Read the model definition and answer for the solid it produces. Units are mm, in the model's axes. A direction names the side the tool comes from. Coordinates: 2 decimals unless noted, no trailing zeros. Loops run counter-clockwise (first coordinate to the right, second up) from the corner with the lowest first, then second, coordinate; pieces in that order, holes last. Notation, with made-up numbers: (-19, 65.5) - (9, 65.5) arc R8 ccw to (9, 78.5) - close; hole circle Ø6 at (79.25, 86). An arc over 180 degrees is marked (long way). One line per question, with ' | ' between items. Start each with the question number.
```python
from build123d import *

# Parameters (mm, degrees)
SKETCH1_W           = 95.25
SKETCH1_H           = 95.25
BOSS_EXTRUDE1_DEPTH = 8.89
SKETCH2_OUTSIDE_W   = 124.25
SKETCH2_OUTSIDE_H   = 124.25
SKETCH2_OUTSIDE_W_2 = 95.25
SKETCH2_OUTSIDE_H_2 = 95.25
SKETCH2_OUTSIDE_R   = 2.38125
CUT_EXTRUDE2_DEPTH  = 9.89
SKETCH3_R           = 6.35
CUT_EXTRUDE3_DEPTH  = 4.445
SKETCH4_R           = 3.3655
CUT_EXTRUDE4_DEPTH  = 5.445


with BuildPart() as part:
    # Sketch1 → Boss-Extrude1 (new body)
    with BuildSketch(Plane.XY):
        Rectangle(SKETCH1_W, SKETCH1_H)
    extrude(amount=BOSS_EXTRUDE1_DEPTH)

    # Sketch2 outside → Cut-Extrude2 (cut, through all)
    with BuildSketch(Plane.XY.offset(8.89)):
        Rectangle(SKETCH2_OUTSIDE_W, SKETCH2_OUTSIDE_H)
        Rectangle(SKETCH2_OUTSIDE_W_2, SKETCH2_OUTSIDE_H_2, mode=Mode.SUBTRACT)
        with Locations((-41.275, 41.275)):
            Circle(SKETCH2_OUTSIDE_R)
        with Locations((41.275, 41.275)):
            Circle(SKETCH2_OUTSIDE_R)
        with Locations((41.275, -41.275)):
            Circle(SKETCH2_OUTSIDE_R)
        with Locations((-41.275, -41.275)):
            Circle(SKETCH2_OUTSIDE_R)
    extrude(amount=-CUT_EXTRUDE2_DEPTH, mode=Mode.SUBTRACT)

    # Sketch3 → Cut-Extrude3 (cut)
    with BuildSketch(Plane.XY.offset(8.89)):
        with Locations((24.765, 29.845)):
            Circle(SKETCH3_R)
    extrude(amount=-CUT_EXTRUDE3_DEPTH, mode=Mode.SUBTRACT)

    # Sketch4 → Cut-Extrude4 (cut, through all)
    with BuildSketch(Plane.XY.offset(4.445)):
        with Locations((24.765, 29.845)):
            Circle(SKETCH4_R)
    extrude(amount=-CUT_EXTRUDE4_DEPTH, mode=Mode.SUBTRACT)


solid = part.part
```
1) Given pin 1 Ø4 at (x, y) = (41.275, 41.275) entering from +Z, flat-ended and moving along its own axis, determine where the tip first touches the part or whether it passes through.
2) Which of the six approach directions +Z, -Z, +X, -X, +Y, -Y give full straight-line access (tool end or side, diameter ignored) to faces 1 (the cylindrical face through (-39.075, 40.363, 4.507)), 2 (the flat face through (27, 27, 4.445))?
3) The mould has two halves that part along Y. Classify faces 3 (the cylindrical face through (23.388, 23.646, 6.699)), 4 (the flat face through (-1, 1, 0)), 5 (the flat face through (-1, 47.625, 4)): released by +Y, released by -Y, zero draft, split by the parting line, or undercut.
4) The part is cut by section A-A on z = 7.5. Count the separate pieces of the cut face and the enclosed holes in it, and give its area (3 significant figures).
5) The part is cut by section B-B on y = 31.5. Write down the section's boundary in (x, z) (3 decimals), and give its area (3 significant figures).
6) Find the intervals of material crossed by line 1 along X through (y, z) = (33, 7.75) (3 decimals); line 2 along Y through (x, z) = (26, 2) (3 decimals), in increasing order. Write a range as from..to.
Answer below:
1) pin 1: through
2) face 1: +Z, -Z | face 2: +Z
3) face 3: undercut | face 4: zero draft | face 5: released by +Y
4) separate pieces: 1 | enclosed holes: 5 | area: 8,870 mm2
5) outline: (-47.625, 0) - (21.835, 0) - (21.835, 4.445) - (18.634, 4.445) - (18.634, 8.89) - (-47.625, 8.89) - close; (27.695, 0) - (47.625, 0) - (47.625, 8.89) - (30.896, 8.89) - (30.896, 4.445) - (27.695, 4.445) - close | area: 766 mm2
6) line 1: -47.625..19.254, 30.276..47.625 | line 2: -47.625..26.714, 32.976..47.625
